Source: CAD feature listing. Evaluate the final solid. Frame: model axes, mm. Round coordinates to 2 decimals unless told otherwise and drop trailing zeros. Write each loop counter-clockwise with the first axis right and the second up, starting at its lowest first coordinate (ties: lowest second). Pieces come first, ordered by that corner, then holes. Notation, with made-up numbers: (63.25, 20.25) -> (76.25, 20.25) arc R19 ccw to (76.25, 53.25) -> close; hole circle Ø6 at (64.25, 32.25). An arc over 180 degrees is marked (long way). Put each result on its own line as item: value.
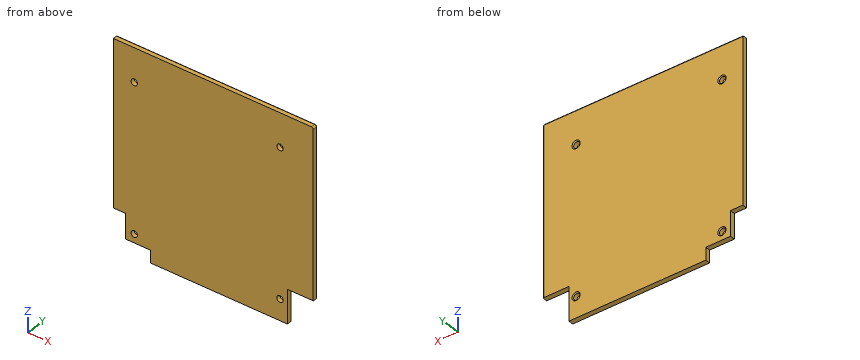
```python
from build123d import *

# Parameters (mm, degrees)
SKETCH1_R           = 1.85
BOSS_EXTRUDE1_DEPTH = 2
CHAMFER2_SIZE       = 1.5
CUT_EXTRUDE2_START  = -2
SKETCH1_4_R         = 2.6
SKETCH1_4_R_2       = 1.85
CUT_EXTRUDE2_DEPTH  = 3.25
FILLET1_R           = 0.75


with BuildPart() as part:
    # Sketch1 → Boss-Extrude1 (new, symmetric)
    with BuildSketch(Plane(origin=(0, 0, 0), x_dir=(1, 0, 0), z_dir=(0, 1, 0))):
        with BuildLine():
            Line((-66.2, 46.15), (-76.2, 46.15))
            Line((-76.2, 46.15), (-76.2, -86.25))
            Line((-76.2, -86.25), (84.75, -86.25))
            ThreePointArc((84.75, -86.25), (85.810660172, -85.810660172), (86.25, -84.75))
            Line((86.25, -84.75), (86.25, 49.08))
            Line((86.25, 49.08), (65.15, 49.08))
            Line((65.15, 49.08), (65.15, 76.2))
            Line((65.15, 76.2), (-46.15, 76.2))
            Line((-46.15, 76.2), (-46.15, 66.2))
            Line((-46.15, 66.2), (-66.2, 66.2))
            Line((-66.2, 66.2), (-66.2, 46.15))
        make_face()
        with Locations(Location((-59.25, 59.25, 0), (0, 0, 270))):
            Circle(SKETCH1_R, mode=Mode.SUBTRACT)
        with Locations(Location((-59.25, -59.25, 0), (0, 0, 270))):
            Circle(SKETCH1_R, mode=Mode.SUBTRACT)
        with Locations(Location((59.25, -59.25, 0), (0, 0, 270))):
            Circle(SKETCH1_R, mode=Mode.SUBTRACT)
        with Locations(Location((59.25, 59.25, 0), (0, 0, 270))):
            Circle(SKETCH1_R, mode=Mode.SUBTRACT)
    extrude(amount=BOSS_EXTRUDE1_DEPTH, both=True)

    # Chamfer2
    chamfer2_edges = [part.edges().sort_by_distance(p)[0] for p in [
        (-59.25, 2, -61.1),
        (59.25, 2, -61.1),
        (59.25, 2, 57.4),
        (-59.25, 2, 57.4),
    ]]
    chamfer(chamfer2_edges, length=CHAMFER2_SIZE)

    # Sketch1<4> → Cut-Extrude2 (cut)
    # profile 1 of 4: a face of its own
    with BuildSketch(Plane(origin=(0, 0, 0), x_dir=(1, 0, 0), z_dir=(0, 1, 0)).offset(CUT_EXTRUDE2_START)):
        with Locations(Location((-59.25, 59.25, 0), (0, 0, 270))):
            Circle(SKETCH1_4_R)
        with Locations((-59.25, 59.25)):
            Circle(SKETCH1_4_R_2, mode=Mode.SUBTRACT)
    # profile 2 of 4: a face of its own
    with BuildSketch(Plane(origin=(0, 0, 0), x_dir=(1, 0, 0), z_dir=(0, 1, 0)).offset(CUT_EXTRUDE2_START)):
        with Locations(Location((-59.25, -59.25, 0), (0, 0, 270))):
            Circle(SKETCH1_4_R)
        with Locations((-59.25, -59.25)):
            Circle(SKETCH1_4_R_2, mode=Mode.SUBTRACT)
    # profile 3 of 4: a face of its own
    with BuildSketch(Plane(origin=(0, 0, 0), x_dir=(1, 0, 0), z_dir=(0, 1, 0)).offset(CUT_EXTRUDE2_START)):
        with Locations(Location((59.25, -59.25, 0), (0, 0, 270))):
            Circle(SKETCH1_4_R)
        with Locations((59.25, -59.25)):
            Circle(SKETCH1_4_R_2, mode=Mode.SUBTRACT)
    # profile 4 of 4: a face of its own
    with BuildSketch(Plane(origin=(0, 0, 0), x_dir=(1, 0, 0), z_dir=(0, 1, 0)).offset(CUT_EXTRUDE2_START)):
        with Locations(Location((59.25, 59.25, 0), (0, 0, 270))):
            Circle(SKETCH1_4_R)
        with Locations((59.25, 59.25)):
            Circle(SKETCH1_4_R_2, mode=Mode.SUBTRACT)
    extrude(amount=CUT_EXTRUDE2_DEPTH, mode=Mode.SUBTRACT)

    # Fillet1
    fillet1_edges = [part.edges().sort_by_distance(p)[0] for p in [
        (86.25, 2, 17.835),
        (4.275, 2, 86.25),
        (85.810660172, 2, 85.810660172),
    ]]
    fillet(fillet1_edges, radius=FILLET1_R)


solid = part.part
```
Q1. Cut plane A-A on z = 59.25. Output: boundary loops of the cut face in (x, y), and give its area (3 significant figures).
Ans:
outline: (-76.2, -2) -> (-61.85, -2) -> (-61.85, 1.25) -> (-62.6, 2) -> (-76.2, 2) -> close; (-56.65, -2) -> (56.65, -2) -> (56.65, 1.25) -> (55.9, 2) -> (-55.9, 2) -> (-56.65, 1.25) -> close; (61.85, -2) -> (86.25, -2) -> (86.25, 1.25) arc R0.75 ccw to (85.5, 2) -> (62.6, 2) -> (61.85, 1.25) -> close
area: 607 mm^2
Q2. Cut plane D-D on z = -59.25. Output: boundary loops of the cut face in (x, y), and give its area (3 significant figures).
Ans:
outline: (-66.2, -2) -> (-61.85, -2) -> (-61.85, 1.25) -> (-62.6, 2) -> (-66.2, 2) -> close; (-56.65, -2) -> (56.65, -2) -> (56.65, 1.25) -> (55.9, 2) -> (-55.9, 2) -> (-56.65, 1.25) -> close; (61.85, -2) -> (65.15, -2) -> (65.15, 2) -> (62.6, 2) -> (61.85, 1.25) -> close
area: 483 mm^2
Q3. Material intervals for line 1 (Z direction, x = -59.5, y = 1.15); line 2 (X direction, y = -0.85, z = 59.25); line 3 (X direction, y = -1.2, z = -59.25), sorted ascending. Write a range as [from, to].
Ans:
line 1: z = [-66.2, -61.84], [-56.66, 56.66], [61.84, 86.25]
line 2: x = [-76.2, -61.85], [-56.65, 56.65], [61.85, 86.25]
line 3: x = [-66.2, -61.85], [-56.65, 56.65], [61.85, 65.15]
Q4. Cut plane C-C on y = -0.65. Output: boundary loops of the cut face in (x, z).
Ans:
outline: (-76.2, -46.15) -> (-66.2, -46.15) -> (-66.2, -66.2) -> (-46.15, -66.2) -> (-46.15, -76.2) -> (65.15, -76.2) -> (65.15, -49.08) -> (86.25, -49.08) -> (86.25, 84.75) arc R1.5 ccw to (84.75, 86.25) -> (-76.2, 86.25) -> close; hole circle Ø5.2 at (-59.25, -59.25); hole circle Ø5.2 at (-59.25, 59.25); hole circle Ø5.2 at (59.25, -59.25); hole circle Ø5.2 at (59.25, 59.25)
Q5. Cut plane B-B on x = -59.25. Output: boundary loops of the cut face in (y, z), and give its area (3 significant figures).
Ans:
outline: (-2, -66.2) -> (2, -66.2) -> (2, -62.6) -> (1.25, -61.85) -> (-2, -61.85) -> close; (-2, -56.65) -> (1.25, -56.65) -> (2, -55.9) -> (2, 55.9) -> (1.25, 56.65) -> (-2, 56.65) -> close; (-2, 61.85) -> (1.25, 61.85) -> (2, 62.6) -> (2, 85.5) arc R0.75 ccw to (1.25, 86.25) -> (-2, 86.25) -> close
area: 567 mm^2
Q6. Pin query (flat end, axial travel): pin 1 (1.2 mm diameter, centred on x = -72.5, y = 0, fed in from -Z); pin 2 (1.2 mm diameter, centred on y = -0.5, z = -56, fed in from -X); pin 3 (2 mm diameter, centred on y = 0.5, z = -69.5, fed in from -X). Return the tip coordinate at first contact, or that it passes through.
Ans:
pin 1: stops at z = -46.15
pin 2: stops at x = -66.2
pin 3: stops at x = -46.15
